Autodesk Inventor part; units mm, degrees
ref_plane "YZ Plane" through (0, 0, 0) normal (1, 0, 0) x (0, 1, 0)
ref_plane "XZ Plane" through (0, 0, 0) normal (0, 1, 0) x (-1, 0, 0)
ref_plane "XY Plane" through (0, 0, 0) normal (0, 0, 1) x (1, 0, 0)
sketch "Sketch1" plane through (0, 0, 0) normal (0, 1, 0) x (-1, 0, 0)
  line L0 (0, -21.955) -> (0, -12.2) construction
  line L1 (13.6, -21.955) -> (13.6, -12.2) construction
  line L2 (-11, -20.9069) -> (-11, 21.1673) construction
  line L3 (16.0254, 0) -> (-21.0399, 0) construction
  line L4 (13.6, -6.2) -> (0, -6.2)
  line L5 (13.6, 6.2) -> (0, 6.2)
  line L6 (6.8, -14.862) -> (6.8, 12.9569) construction
  line L7 (13.6, -6.2) -> (13.6, 6.2)
  line L8 (13.6, 6.2) -> (13.6, 12.2)
  line L9 (0, -6.2) -> (0, 6.2)
  line L10 (0, 6.2) -> (0, 12.2)
  line L11 (13.6, -12.2) -> (0, -12.2)
  line L12 (13.6, 12.2) -> (0, 12.2)
  line L13 (13.6, -12.2) -> (13.6, -6.2)
  line L14 (0, -12.2) -> (0, -6.2)
  line L15 (13.6, 12.2) -> (13.6, 20.1192) construction
  line L16 (0, 12.2) -> (0, 20.7166) construction
  line L17 (9.8, -9.2) -> (3.8, -9.2) construction
  line L18 (3.8, -9.2) -> (3.8, 9.2) construction
  line L19 (3.8, 9.2) -> (9.8, 9.2) construction
  line L20 (9.8, 9.2) -> (9.8, -9.2) construction
  circle A0 centre (6.8, 0) radius 4.25
  point P0 (0, 0)
  dimension "d0" = 24.6
  dimension "d1" = 12.4
  dimension "d2" = 6
  dimension "d4" = 6
  dimension "d17" = 8.5
  dimension "d21" = 6.8
extrude "Extrusion1" add sketch "Sketch1" along normal blind 4 contours L13 L11 L14 L4 | L5 L10 L12 L8
extrude "Extrusion2" add sketch "Sketch1" along normal blind 4 contours L4 L9 L5 L7 | A0
fillet "Fillet1" radius 2 4 edges at (0, 2, 12.2) (-13.6, 2, 12.2) (-13.6, 2, -12.2) (0, 2, -12.2)
extrude "Extrusion3" add sketch "Sketch1" along normal blind 11 contours A0
fillet "Fillet2" radius 0.5 9 edges at (-2.55, 11, 0) (0, 4, 0) (-13.6, 4, 0) (-0.5858, 4, -11.6142) (-6.8, 4, -12.2) (-13.0142, 4, -11.6142) (-0.5858, 4, 11.6142) (-6.8, 4, 12.2) (-13.0142, 4, 11.6142)
sketch "Sketch3" plane through (0, 4, 0) normal (0, 1, 0) x (1, 0, 0)
  point P0 (0, 0)
  point P1 (-9.8, -9.2)
  point P2 (-3.8, -9.2)
  point P3 (-9.8, 9.2)
  point P4 (-3.8, 9.2)
hole "Hole2" at (-9.8, 4, 9.2) at (-3.8, 4, 9.2) at (-9.8, 4, -9.2) at (-3.8, 4, -9.2) direction (0, -1, 0) diameter 2.3 depth 6.5 countersink diameter 4.5 countersink angle 90
properties part number "LegPin_v1"
Work out the finished part from the listing and answer in its coordinate system (mm). Give positions to 0.01 mm unless a question says otherwise; leave off trailing zeros. Order: outer loops, then holes, each group sorted by start corner. A loop starts at its lowest first (then second) coordinate and runs counter-clockwise, first axis right, second up. Notation, with made-up numbers: (19, -27.75) - (49, -27.75) arc R28 cw to (49, 7.25) - close; hole circle Ø6 at (-14.5, 25.5). An arc over 180 degrees is marked (long way). Answer as CSV lines item,"result". Start each with the question number.
Q1. The mould has two halves that part along Z. Classify faces 1 (the face through (-2.5, 4, -2.4)), 2 (the face through (-3.36, 1.43, -8.138)), 3 (the face through (-13, 1.77, -11.63)), 4 (the face through (-3.1, 1.43, 8.29)): +Z half, -Z half, draft (parallel to the pull), parting line (faces both ways), or undercut.
Q2. Given pin 1 Ø3.5 at (x, z) = (-3.8, -9.2) entering from +Y; pin 2 Ø1 at (x, y) = (-4.5, 6.5) entering from +Z; pin 3 Ø3 at (x, z) = (-9.8, 9.2) entering from +Y, each flat-ended and moving along its own axis, determine where each tip first touches the part or whether it passes through.
Q3. The part is cut by section C-C (y = 5.25). Write down the section's boundary in (x, z), then the cut area to 3 significant figures.
Q4. The part is cut by section D-D (z = 6). Write down the section's boundary in (x, y).
Q5. The part is cut by section B-B (y = 1.5). Write down the section's boundary in (x, z).
Q6. The part is cut by section A-A (z = -9.2). Write down the section's boundary in (x, y).
Q7. Find the intervals of material crossed by L1, parallel to X at y = 1.4, z = 9.2; L2, parallel to Z at x = -9.8, y = 1.4; L3, parallel to Y at x = -13, z = -1, in increasing order. Write a range as [from, to].
Check result:
1,face 1,"draft"
1,face 2,"undercut"
1,face 3,"-Z half"
1,face 4,"undercut"
2,pin 1,"stops at y = 3.5"
2,pin 2,"stops at z = 3.85"
2,pin 3,"stops at y = 3.25"
3,outline,"circle Ø8.5 at (-6.8, 0)"
3,area,"56.7 mm²"
4,outline,"(-13.6, 0) - (0, 0) - (0, 3.5) arc R0.5 ccw to (-0.5, 4) - (-13.1, 4) arc R0.5 ccw to (-13.6, 3.5) - close"
5,outline,"(-13.6, -10.2) arc R2 ccw to (-11.6, -12.2) - (-2, -12.2) arc R2 ccw to (0, -10.2) - (0, 10.2) arc R2 ccw to (-2, 12.2) - (-11.6, 12.2) arc R2 ccw to (-13.6, 10.2) - close; hole circle Ø2.3 at (-9.8, -9.2); hole circle Ø2.3 at (-9.8, 9.2); hole circle Ø2.3 at (-3.8, -9.2); hole circle Ø2.3 at (-3.8, 9.2)"
6,outline,"(-13.6, 0) - (-10.95, 0) - (-10.95, 2.9) - (-12.05, 4) - (-13.1, 4) arc R0.5 ccw to (-13.6, 3.5) - close; (-8.65, 0) - (-4.95, 0) - (-4.95, 2.9) - (-6.05, 4) - (-7.55, 4) - (-8.65, 2.9) - close; (-2.65, 0) - (0, 0) - (0, 3.5) arc R0.5 ccw to (-0.5, 4) - (-1.55, 4) - (-2.65, 2.9) - close"
7,L1,"x = [-13.6, -10.95], [-8.65, -4.95], [-2.65, 0]"
7,L2,"z = [-12.2, -10.35], [-8.05, 8.05], [10.35, 12.2]"
7,L3,"y = [0, 4]"
